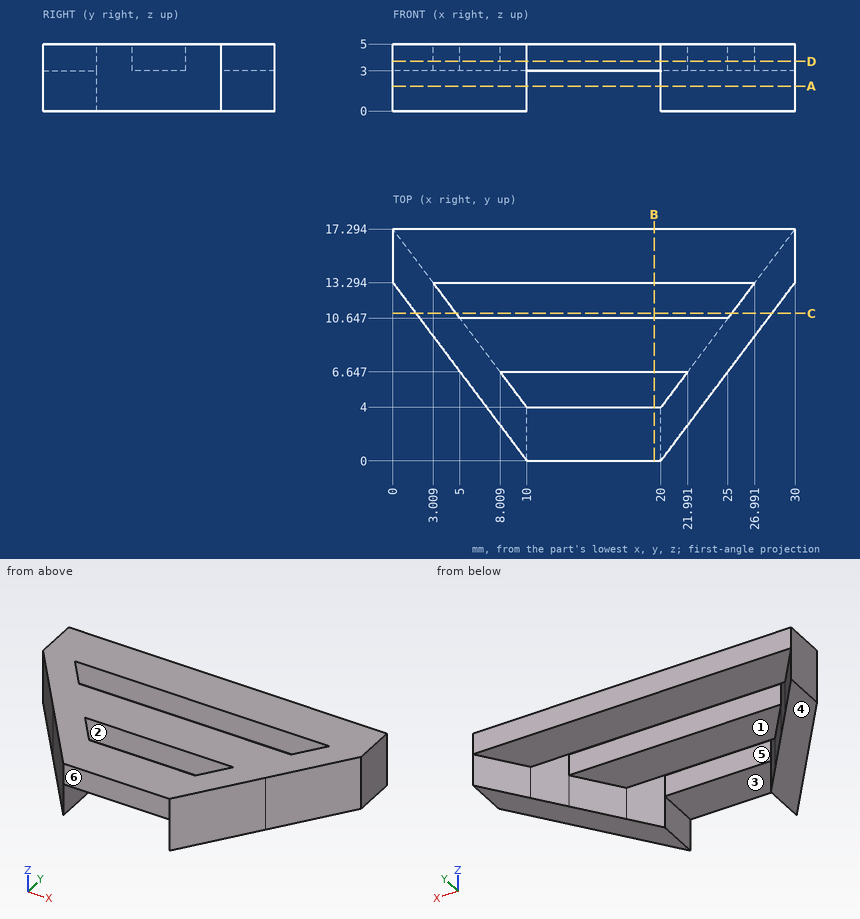
Can you work these out from the drawing? Everything is in mm from the part's minimum corner. A direction names the side the tool comes from. Give positions to 0.01 mm unless a question says otherwise; leave off trailing zeros. Loops run counter-clockwise (first coordinate to the right, second up) from the corner with the lowest first, then second, coordinate; pieces in that order, holes last. Notation, with made-up numbers: (-14.75, 82) - (14.25, 82) arc R29 ccw to (14.25, 119) - close; hole circle Ø4 at (65, 84). An arc over 180 degrees is marked (long way). Answer as a JSON object with one key per item and string values.
Q1. Imagine slicing it at C-C on y = 11. Write out the boundary of the cut face in (x, z), plus the area to 3 significant figures.
Geometry says:
{"outline": "(1.73, 0) - (4.73, 0) - (4.73, 5) - (1.73, 5) - close; (25.27, 0) - (28.27, 0) - (28.27, 5) - (25.27, 5) - close", "area": "30.1 mm²"}
Q2. Imagine slicing it at D-D on z = 3.7. Write out the boundary of the cut face in (x, y).
Geometry says:
{"outline": "(0, 13.29) - (10, 0) - (20, 0) - (30, 13.29) - (30, 17.29) - (0, 17.29) - close; hole (3.01, 13.29) - (5, 10.65) - (25, 10.65) - (26.99, 13.29) - close; hole (8.01, 6.65) - (10, 4) - (20, 4) - (21.99, 6.65) - close"}
Q3. Will these pins go through, and if not, where does the flat tip stop? P1, Ø1.5, axis at y = 12, z = 4, coming from the +X side; P2, Ø2, axis at x = 13, y = 9, coming from the -Z side; P3, Ø0.9, axis at y = 2, z = 1.5, coming from the -X side; P4, Ø2, axis at x = 11.5, z = 4, coming from the -Y side.
Geometry says:
{"P1": "x = 29.59", "P2": "z = 3", "P3": "x = 8.16", "P4": "y = 0"}
Q4. If I drill on L1, parallel to Y at x = 10.5, z = 3.5; L2, parallel to Z at x = 16, y = 7.5; L3, parallel to X at y = 12.5, z = 2.6, over which ranges is the centre line in solid material (lowest first)?
Geometry says:
{"L1": "0 to 4, 6.65 to 10.65, 13.29 to 17.29", "L2": "3 to 5", "L3": "0.6 to 3.61, 26.39 to 29.4"}
Q5. Which directions (+Z, -Z, +X, -X, +Y, -Y) give clear straight access to the entire face, cutting with the end or side of a thin tool? Please do the marked faces 1, 2 and 3.
Geometry says:
{"face 1": "-Z, +Y", "face 2": "+Z, -Z", "face 3": "-Z, +Y, -Y"}
Q6. Imagine slicing it at B-B on x = 19.5. Write out the boundary of the cut face in (y, z).
Geometry says:
{"outline": "(0, 3) - (4, 3) - (4, 5) - (0, 5) - close; (6.65, 3) - (10.65, 3) - (10.65, 5) - (6.65, 5) - close; (13.29, 3) - (17.29, 3) - (17.29, 5) - (13.29, 5) - close"}
Q7. Imagine slicing it at A-A on z = 1.85. Write out the boundary of the cut face in (x, y).
Geometry says:
{"outline": "(0, 13.29) - (10, 0) - (10, 4) - (0, 17.29) - close; (20, 0) - (30, 13.29) - (30, 17.29) - (20, 4) - close"}
Q8. If we mould it in two halves opening along Y, with no side actions, what happens to the marked faces 4, 5 and 6? For each: pulls with the +Y half, pulls with the -Y half, needs draft (parallel to the pull), parting line crosses it, or undercut.
Geometry says:
{"face 4": "needs draft", "face 5": "undercut", "face 6": "pulls with the -Y half"}
